Autodesk Inventor part; units mm, degrees
ref_plane "YZ Plane" through (0, 0, 0) normal (1, 0, 0) x (0, 1, 0)
ref_plane "XZ Plane" through (0, 0, 0) normal (0, 1, 0) x (-1, 0, 0)
ref_plane "XY Plane" through (0, 0, 0) normal (0, 0, 1) x (1, 0, 0)
sketch "Sketch1" plane through (0, 0, 0) normal (0, 0, 1) x (1, 0, 0)
  circle A0 centre (60, -12) radius 5
  line L0 (0, 0) -> (0, 90) construction
  circle A1 centre (-60, -12) radius 5
  line L1 (46, -110) -> (-46, -110)
  line L2 (-46, -110) -> (-46, -110)
  line L3 (-46, -110) -> (-81, -110)
  line L4 (-81, 90) -> (88, 90)
  line L5 (88, 90) -> (88, 190)
  line L6 (88, 190) -> (156, 190)
  line L7 (156, 190) -> (156, -110)
  line L8 (156, -110) -> (46, -110)
  line L9 (46, -110) -> (46, -110)
  line L10 (-81, -110) -> (-81, 90)
  circle A2 centre (30, 67) radius 5
  circle A3 centre (-30, 67) radius 5
  circle A4 centre (60, -58) radius 5
  circle A5 centre (-60, -58) radius 5
  circle A6 centre (-61, -85) radius 5.5
  circle A7 centre (140, -80) radius 5.5
  circle A8 centre (137, 165) radius 5.5
  circle A9 centre (-61, 40) radius 5.5
  line L11 (-60, -58) -> (-60, -78)
  point P0 (0, -110)
  dimension "d82" = 10
  dimension "d83" = 60
  dimension "d86" = 110
  dimension "d87" = 90
  dimension "d88" = 92
  dimension "d90" = 300
  dimension "d91" = 200
  dimension "d92" = 35
  dimension "d93" = 68
  dimension "d94" = 100
  dimension "d95" = 237
  dimension "d96" = 79
  dimension "d98" = 60
  dimension "d100" = 46
  dimension "d101" = 11
  dimension "d102" = 140
  dimension "d103" = 80
  dimension "d104" = 3
  dimension "d105" = 165
  dimension "d106" = 61
  dimension "d107" = 85
  dimension "d108" = 40
  dimension "d136" = 12
  dimension "d139" = 20
extrude "Extrusion1" add sketch "Sketch1" along normal blind 10
thread "Thread1"
thread "Thread2"
thread "Thread3"
thread "Thread4"
properties part number "SUPPORT MAIN FRAME MOTOR-BALL SCREW-REV-B" material "Steel"
The listing builds one solid part. Answer for the finished solid, in the listing's coordinates (mm). A direction names the side the tool comes from. Give positions to 0.01 mm unless a question says otherwise; leave off trailing zeros. Order: outer loops, then holes, each group sorted by start corner. A loop starts at its lowest first (then second) coordinate and runs counter-clockwise, first axis right, second up. Notation, with made-up numbers: (-2.75, -26) - (16.25, -26) arc R24 cw to (16.25, -6) - close; hole circle Ø3 at (12.5, -9). An arc over 180 degrees is marked (long way). Use one line per item in the form item = value.
1) Find section A-A on x = 30. Determine the outline of the cut face in (y, z).
Verdict:
outline = (-110, 0) - (62, 0) - (62, 10) - (-110, 10) - close; (72, 0) - (90, 0) - (90, 10) - (72, 10) - close
2) Find section D-D on y = 67. Determine the outline of the cut face in (x, z).
Verdict:
outline = (-81, 0) - (-35, 0) - (-35, 10) - (-81, 10) - close; (-25, 0) - (25, 0) - (25, 10) - (-25, 10) - close; (35, 0) - (156, 0) - (156, 10) - (35, 10) - close
3) Consider probe 1 along Y at (x, z) = (64.5, 4); probe 2 along X at (y, z) = (-15.5, 9.5); probe 3 along X at (y, z) = (-10, 7). Determine where each line is inside the solid, lowest interval first. Write a range as [from, to].
Verdict:
probe_1 = [-110, -60.18], [-55.82, -14.18], [-9.82, 90]
probe_2 = [-81, -63.57], [-56.43, 56.43], [63.57, 156]
probe_3 = [-81, -64.58], [-55.42, 55.42], [64.58, 156]
4) Find section B-B on y = 165. Determine the outline of the cut face in (x, z), and give its area (3 significant figures).
Verdict:
outline = (88, 0) - (131.5, 0) - (131.5, 10) - (88, 10) - close; (142.5, 0) - (156, 0) - (156, 10) - (142.5, 10) - close
area = 570 mm^2
5) Find section C-C on z = 4.75. Give the number of separate pieces and of enclosed holes in the cut face, and give its area (3 significant figures).
Verdict:
separate_pieces = 1
enclosed_holes = 10
area = 53,300 mm^2
6) The mould has two halves that part along X. Classify faces 3 (the cylindrical face through (59.349, -62.957, 4.93)), 4 (the flat face through (39, -110, 5)), 5 (the flat face through (88, 139, 5)): released by +X, released by -X, zero draft, split by the parting line, or undercut.
Verdict:
face_3 = undercut
face_4 = zero draft
face_5 = released by -X
7) For faces 1 (the flat face through (2, 90, 5)), 2 (the flat face through (36, 9, 0)), determine the directions among +Z, -Z, +X, -X, +Y, -Y from which every point of the face is accessible in a straight line to the end or side of a thin tool.
Verdict:
face_1 = +Z, -Z, -X, +Y
face_2 = -Z, +X, -X, +Y, -Y
8) Each of these flat-tipped pins is pushed along its axis until it touches: pin 1 (14.5 mm diameter, centred on x = 137, y = 165, fed in from -Z); pin 2 (6 mm diameter, centred on y = 123.5, z = 6, fed in from -X). Where does it stop, or does it pass through?
Verdict:
pin_1 = 0
pin_2 = 88
